```python
from build123d import *

# Parameters (mm, degrees)
SCHIZZO1_W                    = 200
SCHIZZO1_H                    = 20
ESTRUSIONE_ESTRUSIONE1_DEPTH  = 25
SCHIZZO2_R                    = 2.25
TAGLIO_ESTRUSIONE1_DEPTH      = 141.400046302
SCHIZZO4_W                    = 2.020725942
SCHIZZO4_H                    = 10
SCHIZZO4_W_2                  = 2.598076211
SCHIZZO4_W_3                  = 3.175426481
TAGLIO_ESTRUSIONE2_DEPTH      = 1
SCHIZZO7_W                    = 15
SCHIZZO7_H                    = 5.5
TAGLIO_ESTRUSIONE3_DEPTH      = 141.400046302
SMUSSO1_SIZE                  = 1.5
SMUSSO1_SIZE2                 = 6
SCHIZZO8_W                    = 25
SCHIZZO8_H                    = 2.5
TAGLIO_ESTRUSIONE4_DEPTH      = 13
SCHIZZO9_W                    = 40
SCHIZZO9_H                    = 2.5
TAGLIO_ESTRUSIONE5_DEPTH      = 141.400046302
SCHIZZO10_W                   = 7
SCHIZZO10_H                   = 3
ESTRUSIONE_ESTRUSIONE5_DEPTH  = 4
SMUSSO2_SIZE                  = 4
SCHIZZO11_W                   = 2.5
SCHIZZO11_H                   = 8
TAGLIO_ESTRUSIONE6_DEPTH      = 141.400046302
SCHIZZO12_W                   = 6.5
SCHIZZO12_H                   = 6.5
TAGLIO_ESTRUSIONE7_DEPTH      = 4
SCHIZZO13_W                   = 9
SCHIZZO13_H                   = 10
ESTRUSIONE_ESTRUSIONE9_DEPTH  = 9
SCHIZZO14_W                   = 13
SCHIZZO14_H                   = 14
ESTRUSIONE_ESTRUSIONE10_DEPTH = 3.5
SMUSSO3_SIZE                  = 9
SMUSSO3_SIZE2                 = 4
SMUSSO4_SIZE                  = 4
SMUSSO4_SIZE2                 = 9
SCHIZZO16_R                   = 2.25
TAGLIO_ESTRUSIONE8_DEPTH      = 141.17038757
SCHIZZO17_R                   = 4
TAGLIO_ESTRUSIONE9_DEPTH      = 5


with BuildPart() as part:
    # Schizzo1 → Estrusione-Estrusione1 (new body)
    with BuildSketch(Plane.XY):
        with Locations((36.701035116, 4.318421053)):
            Rectangle(SCHIZZO1_W, SCHIZZO1_H)
    extrude(amount=ESTRUSIONE_ESTRUSIONE1_DEPTH)

    # Schizzo2 → Taglio-Estrusione1 (cut, through all)
    with BuildSketch(Plane(origin=(0, 14.318421053, 0), x_dir=(1, 0, 0), z_dir=(0, 1, 0))):
        with Locations(Location((-53.298964884, -15, 0), (0, 0, 270))):
            Circle(SCHIZZO2_R)
        Polygon((-23.80414637, -15.875), (-22.793783399, -15.875), (-22.288601913, -15), (-22.793783399, -14.125), (-23.80414637, -14.125), (-24.309327855, -15), align=None)
        Polygon((-14.999926779, -15), (-15.649445831, -13.875), (-16.948483937, -13.875), (-17.59800299, -15), (-16.948483937, -16.125), (-15.649445831, -16.125), align=None)
        Polygon((-8.505108264, -16.375), (-7.711251644, -15), (-8.505108264, -13.625), (-10.092821504, -13.625), (-10.886678125, -15), (-10.092821504, -16.375), align=None)
    extrude(amount=-TAGLIO_ESTRUSIONE1_DEPTH, mode=Mode.SUBTRACT)

    # Schizzo4 → Taglio-Estrusione2 (cut)
    with BuildSketch(Plane(origin=(0, 14.318421053, 0), x_dir=(1, 0, 0), z_dir=(0, 1, 0))):
        with Locations((-23.298964884, -20)):
            Rectangle(SCHIZZO4_W, SCHIZZO4_H)
        with Locations((-16.298964885, -20)):
            Rectangle(SCHIZZO4_W_2, SCHIZZO4_H)
        with Locations((-9.298964885, -20)):
            Rectangle(SCHIZZO4_W_3, SCHIZZO4_H)
    extrude(amount=-TAGLIO_ESTRUSIONE2_DEPTH, mode=Mode.SUBTRACT)

    # Schizzo7 → Taglio-Estrusione3 (cut, through all)
    with BuildSketch(Plane(origin=(0, 14.318421053, 0), x_dir=(1, 0, 0), z_dir=(0, 1, 0))):
        with Locations((14.788748356, -17.25)):
            Rectangle(SCHIZZO7_W, SCHIZZO7_H)
        with Locations((14.788748356, -7.75)):
            Rectangle(SCHIZZO7_W, SCHIZZO7_H)
    extrude(amount=-TAGLIO_ESTRUSIONE3_DEPTH, mode=Mode.SUBTRACT)

    # Smusso1
    smusso1_edges = [part.edges().sort_by_distance(p)[0] for p in [
        (14.788748356, 14.318421053, 14.5),
        (14.788748356, 14.318421053, 10.5),
    ]]
    smusso1_side = [part.faces().sort_by_distance(p)[0] for p in [
        (38.695689024, 14.318421053, 12.36530447),
    ]]
    chamfer(smusso1_edges, length=SMUSSO1_SIZE, length2=SMUSSO1_SIZE2, reference=smusso1_side[0])

    # Schizzo8 → Taglio-Estrusione4 (cut)
    with BuildSketch(Plane(origin=(0, 14.318421053, 0), x_dir=(1, 0, 0), z_dir=(0, 1, 0))):
        with Locations((49.788748356, -18.75)):
            Rectangle(SCHIZZO8_W, SCHIZZO8_H)
        with Locations((49.788748356, -11.25)):
            Rectangle(SCHIZZO8_W, SCHIZZO8_H)
    extrude(amount=-TAGLIO_ESTRUSIONE4_DEPTH, mode=Mode.SUBTRACT)

    # Schizzo9 → Taglio-Estrusione5 (cut, through all)
    with BuildSketch(Plane(origin=(0, 14.318421053, 0), x_dir=(1, 0, 0), z_dir=(0, 1, 0))):
        with Locations((116.701035116, -8.75)):
            Rectangle(SCHIZZO9_W, SCHIZZO9_H)
    extrude(amount=-TAGLIO_ESTRUSIONE5_DEPTH, mode=Mode.SUBTRACT)

    # Schizzo10 → Estrusione-Estrusione5 (add)
    with BuildSketch(Plane(origin=(0, 14.318421053, 0), x_dir=(1, 0, 0), z_dir=(0, 1, 0))):
        with Locations((133.201035116, -6)):
            Rectangle(SCHIZZO10_W, SCHIZZO10_H)
        with Locations((133.201035116, -11.5)):
            Rectangle(SCHIZZO10_W, SCHIZZO10_H)
    extrude(amount=ESTRUSIONE_ESTRUSIONE5_DEPTH)

    # Smusso2
    smusso2_edges = [part.edges().sort_by_distance(p)[0] for p in [
        (129.701035116, 18.318421053, 11.5),
        (129.701035116, 18.318421053, 6),
    ]]
    chamfer(smusso2_edges, length=SMUSSO2_SIZE - 0.0001)  # a hair under: the kernel refuses the full size

    # Schizzo11 → Taglio-Estrusione6 (cut, through all)
    with BuildSketch(Plane(origin=(0, 14.318421053, 0), x_dir=(1, 0, 0), z_dir=(0, 1, 0))):
        with Locations((99.951035116, -21)):
            Rectangle(SCHIZZO11_W, SCHIZZO11_H)
    extrude(amount=-TAGLIO_ESTRUSIONE6_DEPTH, mode=Mode.SUBTRACT)

    # Schizzo12 → Taglio-Estrusione7 (cut)
    with BuildSketch(Plane(origin=(0, 14.318421053, 0), x_dir=(1, 0, 0), z_dir=(0, 1, 0))):
        with Locations((99.951035116, -20.25)):
            Rectangle(SCHIZZO12_W, SCHIZZO12_H)
    extrude(amount=-TAGLIO_ESTRUSIONE7_DEPTH, mode=Mode.SUBTRACT)

    # Schizzo13 → Estrusione-Estrusione9 (add)
    with BuildSketch(Plane.XY.offset(25)):
        with Locations((29.788748356, -0.681578947)):
            Rectangle(SCHIZZO13_W, SCHIZZO13_H)
    extrude(amount=ESTRUSIONE_ESTRUSIONE9_DEPTH)

    # Schizzo14 → Estrusione-Estrusione10 (add)
    with BuildSketch(Plane.XY.offset(34)):
        with Locations((29.788748356, 1.318421053)):
            Rectangle(SCHIZZO14_W, SCHIZZO14_H)
    extrude(amount=ESTRUSIONE_ESTRUSIONE10_DEPTH)

    # Smusso3
    smusso3_edges = [part.edges().sort_by_distance(p)[0] for p in [
        (34.288748356, 4.318421053, 29.5),
    ]]
    smusso3_side = [part.faces().sort_by_distance(p)[0] for p in [
        (34.288748356, -0.681578947, 29.5),
    ]]
    chamfer(smusso3_edges, length=SMUSSO3_SIZE, length2=SMUSSO3_SIZE2, reference=smusso3_side[0])

    # Smusso4
    smusso4_edges = [part.edges().sort_by_distance(p)[0] for p in [
        (25.288748356, 4.318421053, 29.5),
    ]]
    smusso4_side = [part.faces().sort_by_distance(p)[0] for p in [
        (27.788748356, 4.318421053, 29.5),
    ]]
    chamfer(smusso4_edges, length=SMUSSO4_SIZE, length2=SMUSSO4_SIZE2, reference=smusso4_side[0])

    # Schizzo16 → Taglio-Estrusione8 (cut, through all)
    with BuildSketch(Plane.XY.offset(25)):
        with Locations((-37.648964884, 4.318421053)):
            Circle(SCHIZZO16_R)
        with Locations((79.451035116, 4.318421053)):
            Circle(SCHIZZO16_R)
    extrude(amount=-TAGLIO_ESTRUSIONE8_DEPTH, mode=Mode.SUBTRACT)

    # Schizzo17 → Taglio-Estrusione9 (cut)
    with BuildSketch(Plane.XY.offset(25)):
        with Locations((-37.648964884, 4.318421053)):
            Circle(SCHIZZO17_R)
        with Locations((79.451035116, 4.318421053)):
            Circle(SCHIZZO17_R)
    extrude(amount=-TAGLIO_ESTRUSIONE9_DEPTH, mode=Mode.SUBTRACT)


solid = part.part
```
For this review, take the finished solid that the model builds, in its own axes (mm). A direction names the side the tool comes from. Give positions to 0.01 mm unless a question says otherwise; leave off trailing zeros. Loops run counter-clockwise (first coordinate to the right, second up) from the corner with the lowest first, then second, coordinate; pieces in that order, holes last. Notation, with made-up numbers: M 11,1 L 15,1 A20 ccw 15,16 Z; hole C 84.5,39.5 d9. An arc over 180 degrees is marked long. One line per item, written item: value. Start each with the question number.
Q1. Draft analysis for pull direction Y (two halves, no side actions). For faces 1 (the face through (15, 1, 10.5)), 2 (the face through (32.26, -0.12, 29.44)), 3 (the face through (-33.954, 2.786, 22.535)), state which applies: released by +Y, released by -Y, zero draft, split by the parting line, or undercut.
Q2. Machinability: for faces 4 (the face through (30, 8.318, 36)), 5 (the face through (36.289, 1, 36)), 6 (the face through (81.2, 2.6, 20)), 7 (the face through (100, 7, 17)), 8 (the face through (136.701, 6, 4)), which of the approach directions +Z, -Z, +X, -X, +Y, -Y give a long, thin tool a straight path to every point of the face, cutting with its end or side? Answer none if there is none.
Q3. Clearance check with flat-ended pins moving along their axes: pin 1 Ø4 at (x, y) = (16, 4.5) entering from +Z; pin 2 Ø5 at (x, y) = (-37.65, 4.32) entering from +Z; pin 3 Ø1 at (y, z) = (2.5, 36) entering from -X. State where each tip first meets the part, or that it passes through.
Q4. Add section A-A (y = -1.5). Count the separate pieces of the cut face and the enclosed holes in it, and give its area (3 significant figures).
Q5. Add section B-B (x = 2). Give the boundary of the cut face in (y, z).
Q6. For L1, parallel to Z at x = 56, y = 4.75; L2, parallel to X at y = -0.5, z = 7; L3, parallel to Z at x = 20, y = 8.5, list the stretches that pass through material, from the lowest coordinate up.
Reply:
1. face 1: zero draft
1. face 2: released by +Y
1. face 3: undercut
2. face 4: +Z, +X, -X, +Y
2. face 5: +Z, +X, +Y, -Y
2. face 6: +Z
2. face 7: +Y
2. face 8: +Z, -Z, +X, +Y, -Y
3. pin 1: z = 25
3. pin 2: z = 20
3. pin 3: x = 23.29
4. separate pieces: 1
4. enclosed holes: 6
4. area: 4,790 mm²
5. outline: M -5.68,0 L 14.32,0 L 14.32,25 L -5.68,25 Z
6. L1: 0 to 10, 12.5 to 17.5, 20 to 25
6. L2: -63.3 to 7.29, 22.29 to 136.7
6. L3: 0 to 5, 10.55 to 14.45, 20 to 25
